Here's how the part is built. I have some questions about the finished solid (model axes, mm). Round coordinates to 2 decimals unless told otherwise and drop trailing zeros. Order: outer loops, then holes, each group sorted by start corner. A loop starts at its lowest first (then second) coordinate and runs counter-clockwise, first axis right, second up. Notation, with made-up numbers: M 6,84.5 L 64,84.5 A25 ccw 64,107.5 Z; hole C -35,74.25 d5. An arc over 180 degrees is marked long. Use one line per item in the form item = value. Start each with the question number.
```python
from build123d import *

# Parameters (mm, degrees)
SKETCH1_R           = 1.5875
BOSS_EXTRUDE1_DEPTH = 1.6


with BuildPart() as part:
    # Sketch1 → Boss-Extrude1 (new, symmetric)
    with BuildSketch(Plane.XY):
        with BuildLine():
            Line((-143.274111577, 7.39), (143.274111608, 7.39))
            ThreePointArc((143.274111608, 7.39), (147.74272521, 7.792581352), (152.070006331, 8.978))
            ThreePointArc((152.070006331, 8.978), (161.04800313, -3.115e-06), (152.070000015, -8.977999914))
            ThreePointArc((152.070000015, -8.977999914), (147.755008516, -7.718567431), (143.272000016, -7.389999914))
            Line((143.272000016, -7.389999914), (-143.271999985, -7.389999914))
            ThreePointArc((-143.271999985, -7.389999914), (-147.739885513, -7.802353266), (-152.069999985, -8.977999914))
            ThreePointArc((-152.069999985, -8.977999914), (-161.047999985, 8.6e-08), (-152.069999985, 8.978000086))
            ThreePointArc((-152.069999985, 8.978000086), (-147.743155019, 7.790183335), (-143.274111577, 7.39))
        make_face()
        with Locations((-152.069999985, 8.6e-08)):
            Circle(SKETCH1_R, mode=Mode.SUBTRACT)
        with Locations((152.070003173, 4.3e-08)):
            Circle(SKETCH1_R, mode=Mode.SUBTRACT)
    extrude(amount=BOSS_EXTRUDE1_DEPTH, both=True)


solid = part.part
```
1) If I drill on line 1 (X direction, y = -0.25, z = -0.9); line 2 (X direction, y = 0.75, z = 1.5); line 3 (Y direction, x = -68, z = -1.15), over which ranges is the centre line in solid material (lowest first)?
2) If we section it at A-A on z = 0.5: Write out the boundary of the cut face in (x, y) (1 decimal).
3) Will these pins go through, and if not, where does the flat tip stop? pin 1 Ø1 at (y, z) = (-6.5, -1) entering from -X; pin 2 Ø1.6 at (x, z) = (-49.5, -1) entering from +Y; pin 3 Ø3 at (x, y) = (152.07, 0) entering from -Z.
4) If we section it at B-B on x = 84: Write out the boundary of the cut face in (y, z), then the cut area to 3 significant figures.
Completed:
q1.line_1 = -161.04 to -153.64, -150.5 to 150.5, 153.64 to 161.04
q1.line_2 = -161.02 to -153.47, -150.67 to 150.67, 153.47 to 161.02
q1.line_3 = -7.39 to 7.39
q2.outline = M -152.1,-9 A26 cw -143.3,-7.4 L 143.3,-7.4 A21.4 cw 152.1,-9 A9 ccw 152.1,9 A25.3 cw 143.3,7.4 L -143.3,7.4 A25.2 cw -152.1,9 A9 ccw Z; hole C -152.1,0 d3.2; hole C 152.1,0 d3.2
q3.pin_1 = -158.75
q3.pin_2 = 7.39
q3.pin_3 = through
q4.outline = M -7.39,-1.6 L 7.39,-1.6 L 7.39,1.6 L -7.39,1.6 Z
q4.area = 47.3 mm²
